For this review, take the finished solid that the model builds, in its own axes (mm). A direction names the side the tool comes from. Round coordinates to 2 decimals unless told otherwise and drop trailing zeros. Order: outer loops, then holes, each group sorted by start corner. A loop starts at its lowest first (then second) coordinate and runs counter-clockwise, first axis right, second up. Notation, with made-up numbers: M 72.5,-31 L 99.5,-31 A10 cw 99.5,-16 Z; hole C 3.25,66 d7. An arc over 180 degrees is marked long. Put each result on its own line as item: value.
Autodesk Inventor part; units mm, degrees
ref_plane "YZ Plane" through (0, 0, 0) normal (1, 0, 0) x (0, 1, 0)
ref_plane "XZ Plane" through (0, 0, 0) normal (0, 1, 0) x (-1, 0, 0)
ref_plane "XY Plane" through (0, 0, 0) normal (0, 0, 1) x (1, 0, 0)
sketch "Sketch1" plane through (0, 0, 0) normal (1, 0, 0) x (0, 1, 0)
  line L0 (104.8505, 212.4728) -> (49.4505, 212.4728)
  line L1 (49.4505, 212.4728) -> (49.4505, 172.4728)
  line L2 (49.4505, 122.4728) -> (49.4505, 82.4728)
  line L3 (49.4505, 82.4728) -> (104.8505, 82.4728)
  line L4 (104.8505, 82.4728) -> (104.8505, 137.2728)
  line L5 (104.8505, 137.2728) -> (88.4505, 137.2728)
  line L6 (88.4505, 137.2728) -> (88.4505, 157.6728)
  line L7 (88.4505, 157.6728) -> (104.8505, 157.6728)
  line L8 (104.8505, 212.4728) -> (104.8505, 157.6728)
  line L9 (39.4505, 147.4728) -> (88.4505, 147.4728) construction
  line L10 (39.4505, 172.4728) -> (39.4505, 122.4728)
  line L11 (49.4505, 122.4728) -> (39.4505, 122.4728)
  line L12 (49.4505, 172.4728) -> (39.4505, 172.4728)
  point P0 (0, 0)
  dimension "d0" = 10
  dimension "d3" = 55.4
  dimension "d4" = 130
  dimension "d8" = 20.4
  dimension "d9" = 50
  dimension "d10" = 16.4
extrude "Extrusion1" add sketch "Sketch1" along normal blind 10
equation "\"d0\" = Width"
equation "\"d5\" = Width"
equation "\"Width\" = 10"
properties part number "BackWall" material "ABS Plastic"
(1) Draft analysis for pull direction Z (two halves, no side actions). For faces 1 (the face through (5, 88.45, 147)), 2 (the face through (0, 72, 148)), 3 (the face through (5, 77, 82.473)), state which applies: released by +Z, released by -Z, zero draft, split by the parting line, or undercut.
A:
face 1: undercut
face 2: zero draft
face 3: released by -Z
(2) To check wall thickness, follow L1, parallel to Z at x = 7, y = 99; L2, parallel to Y at x = 6, z = 106. State the ranges of each line that lie inside material, in increasing order.
A:
L1: z = 82.47 to 137.27, 157.67 to 212.47
L2: y = 49.45 to 104.85
(3) For faces 4 (the face through (5, 97, 157.673)), 5 (the face through (5, 45, 172.473)), 6 (the face through (5, 39.45, 148)), 7 (the face through (5, 45, 122.473)), list the 3-axis set-ups (+Z, -Z, +X, -X, +Y, -Y) from which the entire face can be reached by the end or side of a thin tool; tool diameter is ignored.
A:
face 4: +X, -X, +Y
face 5: +Z, +X, -X, -Y
face 6: +Z, -Z, +X, -X, -Y
face 7: -Z, +X, -X, -Y
(4) Add section C-C on z = 96.5. Give the boundary of the cut face in (x, y), then the cut area to 3 significant figures.
A:
outline: M 0,49.45 L 10,49.45 L 10,104.85 L 0,104.85 Z
area: 554 mm2
(5) Add section B-B on x = 4.5. Give the boundary of the cut face in (y, z), then the cut area to 3 significant figures.
A:
outline: M 39.45,122.47 L 49.45,122.47 L 49.45,82.47 L 104.85,82.47 L 104.85,137.27 L 88.45,137.27 L 88.45,157.67 L 104.85,157.67 L 104.85,212.47 L 49.45,212.47 L 49.45,172.47 L 39.45,172.47 Z
area: 7,370 mm2
(6) Insertion check: pin 1 Ø5 at (x, z) = (4.5, 107) entering from -Y; pin 2 Ø3 at (x, z) = (1.5, 152.5) entering from +Y; pin 3 Ø5 at (x, y) = (2.5, 45) entering from -Z. Each pin has a flat end and moves straight along its axis. Give the tip position at first contact, or say it passes through.
A:
pin 1: stops at y = 49.45
pin 2: stops at y = 88.45
pin 3: stops at z = 122.47
(7) Add section D-D on y = 45. Give the boundary of the cut face in (x, z).
A:
outline: M 0,122.47 L 10,122.47 L 10,172.47 L 0,172.47 Z
(8) Add section A-A on y = 91.5. Give the boundary of the cut face in (x, z).
A:
outline: M 0,82.47 L 10,82.47 L 10,137.27 L 0,137.27 Z; M 0,157.67 L 10,157.67 L 10,212.47 L 0,212.47 Z
